Can you work these out from the model? Positions are in its coordinate system, mm. Face numbers are marked on the shaded views. A direction names the side the tool comes from. Give positions to 0.01 mm unless a question says otherwise; leave off trailing zeros.
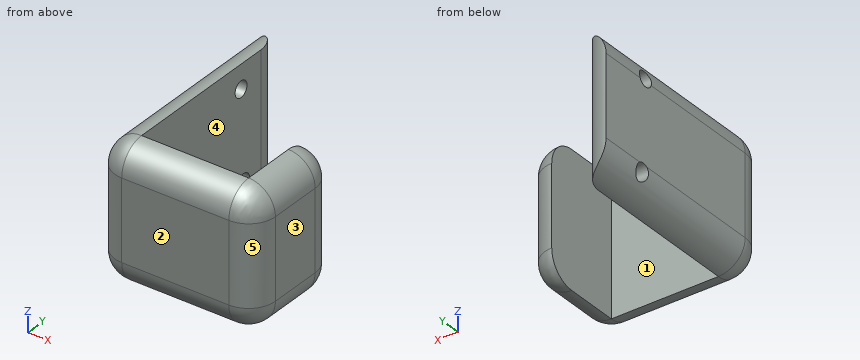
from build123d import *

# Parameters (mm, degrees)
F1_DEPTH    = 25
F2_R        = 4.99999
F3_T1_DEPTH = 40.00001
F3_T3_DEPTH = 45.00001
F3_T6_ANGLE = 90
F4_R        = 4.99999
F5_R        = 4.99999
F6_R        = 4.99999
F7_T1_DEPTH = 27.50001
F7_T3_DEPTH = 25.0000100044
F7_T6_ANGLE = 90
F7_T8_ANGLE = 233.2969892316
F9_R        = 1.5
F10_DEPTH   = 6
F11_DEPTH   = 6


# Not quite as in the source:
# - a fillet or chamfer that OpenCascade refuses, or shapes differently, is made with other operations: its cross-section is extruded or revolved along the edge and cut away or added
# - a fillet or chamfer is up to 0.001 mm smaller than in the source, because OpenCascade refuses the exact size


with BuildPart() as f1:
    # F0 (on Top) → F1 (new body)
    with BuildSketch(Plane.XY):
        Polygon((-55.5160288679, 43.4392371902), (-60.5160288679, 43.4392371902), (-60.5160288679, 3.4392371902), (-30.5160288679, 3.4392371902), (-30.5160288679, 23.4392371902), (-35.5160288679, 23.4392371902), (-35.5160288679, 8.4392371902), (-55.5160288679, 8.4392371902), align=None)
    extrude(amount=F1_DEPTH)

    # F2 (radius 5 in the source; OpenCascade refuses exactly that, so slightly less here)
    f2_edges = [f1.edges().sort_by_distance(p)[0] for p in [
        (-45.516029, 3.439237, 25),
    ]]
    fillet(f2_edges, radius=F2_R)

    # F3: fillet of radius 5 on 1 edges, made by hand

    # F3_s2 → F3_t1 (cut)
    with BuildSketch(Plane.XZ.offset(-35.9392371902)):
        with BuildLine():
            ThreePointArc((-35.5160288679, 25), (-31.980494962, 23.5355339059), (-30.5160288679, 20))
            Line((-30.5160288679, 20), (-30.5160288679, 25))
            Line((-30.5160288679, 25), (-35.5160288679, 25))
        make_face()
    extrude(amount=F3_T1_DEPTH, mode=Mode.SUBTRACT)

    # F3_s4 → F3_t3 (cut)
    with BuildSketch(Plane.XY.offset(-12.5)):
        with BuildLine():
            ThreePointArc((-35.5160288679, 3.4392371902), (-31.980494962, 4.9037032843), (-30.5160288679, 8.4392371902))
            Line((-30.5160288679, 8.4392371902), (-30.5160288679, 3.4392371902))
            Line((-30.5160288679, 3.4392371902), (-35.5160288679, 3.4392371902))
        make_face()
    extrude(amount=F3_T3_DEPTH, mode=Mode.SUBTRACT)

    # F3_s5 → F3_t6 (revolve, cut)
    with BuildSketch(Plane.XY.offset(20.00001)):
        with BuildLine():
            ThreePointArc((-35.5160288679, 3.4392371902), (-31.9804984975, 4.9036997488), (-30.5160288679, 8.4392271902))
            Line((-30.5160288679, 8.4392271902), (-30.5160288679, 3.4392371902))
            Line((-30.5160288679, 3.4392371902), (-35.5160288679, 3.4392371902))
        make_face()
    revolve(axis=Axis((-30.5160288679, 8.4392271902, 20.00001), (-1, 0, 0)), revolution_arc=F3_T6_ANGLE, mode=Mode.SUBTRACT)

    # F4 (radius 5 in the source; OpenCascade refuses exactly that, so slightly less here)
    f4_edges = [f1.edges().sort_by_distance(p)[0] for p in [
        (-30.516029, 15.939237, 0),
    ]]
    fillet(f4_edges, radius=F4_R)

    # F5 (radius 5 in the source; OpenCascade refuses exactly that, so slightly less here)
    f5_edges = [f1.edges().sort_by_distance(p)[0] for p in [
        (-60.516029, 25.939232, 25),
    ]]
    fillet(f5_edges, radius=F5_R)

    # F6 (radius 5 in the source; OpenCascade refuses exactly that, so slightly less here)
    f6_edges = [f1.edges().sort_by_distance(p)[0] for p in [
        (-55.516029, 43.439237, 12.5),
    ]]
    fillet(f6_edges, radius=F6_R)

    # F7: fillet of radius 5 on 4 edges, made by hand

    # F7_s2 → F7_t1 (cut)
    with BuildSketch(Plane.XY.offset(-7.50001)):
        with BuildLine():
            ThreePointArc((-35.5160288679, 23.4392371902), (-31.980494962, 21.9747710962), (-30.5160288679, 18.4392371902))
            Line((-30.5160288679, 18.4392371902), (-30.5160288679, 23.4392371902))
            Line((-30.5160288679, 23.4392371902), (-35.5160288679, 23.4392371902))
        make_face()
    extrude(amount=F7_T1_DEPTH, mode=Mode.SUBTRACT)

    # F7_s4 → F7_t3 (cut)
    with BuildSketch(Plane.YZ.offset(-48.0160288701)):
        with BuildLine():
            ThreePointArc((18.4392371902, 0), (21.9747710962, 1.4644660941), (23.4392371902, 5))
            Line((23.4392371902, 5), (23.4392371902, 0))
            Line((23.4392371902, 0), (18.4392371902, 0))
        make_face()
    extrude(amount=F7_T3_DEPTH, mode=Mode.SUBTRACT)

    # F7_s5 → F7_t6 (revolve, cut)
    with BuildSketch(Plane.YZ.offset(-35.5160188679)):
        with BuildLine():
            ThreePointArc((18.4392371902, 0), (21.9747675606, 1.4644625585), (23.4392371902, 4.99999))
            Line((23.4392371902, 4.99999), (23.4392371902, 0))
            Line((23.4392371902, 0), (18.4392371902, 0))
        make_face()
    revolve(axis=Axis((-35.5160188679, 23.4392371902, 4.99999), (0, -1, 0)), revolution_arc=F7_T6_ANGLE, mode=Mode.SUBTRACT)

    # F7_s7 → F7_t8 (revolve, cut)
    with BuildSketch(Plane(origin=(-32.4130099886, 0, 24.1625626894), x_dir=(0, 1, 0), z_dir=(0.8017442393, 0, -0.5976672777))):
        with BuildLine():
            ThreePointArc((23.4392371902, -5.1918835033), (21.9747710962, -8.7274174092), (18.4392371902, -10.1918835033))
            Line((18.4392371902, -10.1918835033), (23.4392371902, -10.1918835033))
            Line((23.4392371902, -10.1918835033), (23.4392371902, -5.1918835033))
        make_face()
    revolve(axis=Axis((-35.516028868, 23.4392371902, 19.9999999999), (0, 1, 0)), revolution_arc=F7_T8_ANGLE, mode=Mode.SUBTRACT)

    # F9 (on offset) → F10 (cut)
    with BuildSketch(Plane.YZ.offset(-55)):
        with Locations((33.4674492478, 20.548062399)):
            Circle(F9_R)
    extrude(amount=-F10_DEPTH, mode=Mode.SUBTRACT)

    # F9 (on offset) → F11 (cut)
    with BuildSketch(Plane.YZ.offset(-55)):
        with Locations((33.4674492478, 20.548062399)):
            Circle(F9_R)
        with Locations((34.116756171, 3.7890784442)):
            Circle(F9_R)
    extrude(amount=-F11_DEPTH, mode=Mode.SUBTRACT)


solid = f1.part
(1) Please list where these lines run through material, in increasing order: probe 1 along X at (y, z) = (17.5, 11.75); probe 2 along Z at (x, y) = (-57.5, 34); probe 3 along Y at (x, z) = (-39, 8.75).
Returned:
probe 1: x = -60.52 to -55.52, -35.52 to -30.52
probe 2: z = 0.41 to 2.29, 5.28 to 19.15, 21.95 to 24.59
probe 3: y = 3.44 to 8.44
(2) Which directions (+Z, -Z, +X, -X, +Y, -Y) give clear straight access to the entire face, cutting with the end or side of a thin tool? Please do the marked faces 4 and 5.
Returned:
face 4: +Z, -Z, +Y
face 5: +Z, -Z, +X, -Y
(3) Thinking about a two-plate mould opening in X: for the marked faces 1, 2 and 3, which applies, pulls with the +X half, pulls with the -X half, needs draft (parallel to the pull), parting line crosses it, or undercut?
Returned:
face 1: undercut
face 2: needs draft
face 3: pulls with the +X half
(4) Will these pins go through, and if not, where does the flat tip stop? P1, Ø2, axis at y = 18, z = 22, coming from the +X side; P2, Ø4, axis at y = 34.12, z = 3.79, coming from the +X side; P3, Ø6, axis at x = -42, z = 13.5, coming from the +Y side.
Returned:
P1: stops at x = -30.62
P2: stops at x = -55.52
P3: stops at y = 8.44
